Work out the finished part from the listing and answer in its coordinate system (mm). Face numbers are marked on the shaded views. A direction names the side the tool comes from. Coordinates: 2 decimals unless noted, no trailing zeros. Write each loop counter-clockwise with the first axis right and the second up, starting at its lowest first coordinate (ties: lowest second). Pieces come first, ordered by that corner, then holes. Notation, with made-up numbers: (65, 71.5) - (77, 71.5) arc R30 ccw to (77, 95.5) - close; hole circle Ø9 at (45.25, -37). An arc over 180 degrees is marked (long way). Use CSV: the item, a comma, the result in double quotes. Start each with the question number.
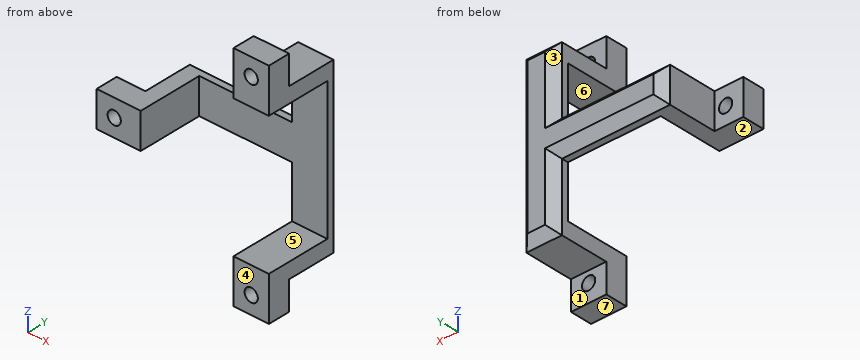
from build123d import *

# Parameters (mm, degrees)
IZIM1_W                       = 10
IZIM1_H                       = 8
IZIM1_R                       = 1.5
Y_KSEKLIK_EKSTR_ZYON1_DEPTH   = 5
IZIM1_W_2                     = 8
IZIM1_H_2                     = 10
Y_KSEKLIK_EKSTR_ZYON1_2_DEPTH = 5
Y_KSEKLIK_EKSTR_ZYON1_3_DEPTH = 5
IZIM2_W                       = 3.5
IZIM2_H                       = 8
IZIM2_W_2                     = 8
IZIM2_H_2                     = 3.5
Y_KSEKLIK_EKSTR_ZYON2_DEPTH   = 13
IZIM3_W                       = 8
IZIM3_H                       = 3.5
Y_KSEKLIK_EKSTR_ZYON3_DEPTH   = 29
IZIM4_W                       = 8
IZIM4_H                       = 3.5
Y_KSEKLIK_EKSTR_ZYON4_DEPTH   = 11.75
IZIM5_W                       = 8
IZIM5_H                       = 3.5
Y_KSEKLIK_EKSTR_ZYON5_DEPTH   = 11.75
PAH1_SIZE                     = 2


with BuildPart() as part:
    # izim1 → Y_kseklik-Ekstr_zyon1 (new body)
    with BuildSketch(Plane(origin=(0, 0, 0), x_dir=(1, 0, 0), z_dir=(0, 1, 0))):
        with Locations((-30, 0)):
            Rectangle(IZIM1_W, IZIM1_H)
        with Locations(Location((-31, 0, 0), (0, 0, 270))):
            Circle(IZIM1_R, mode=Mode.SUBTRACT)
    extrude(amount=Y_KSEKLIK_EKSTR_ZYON1_DEPTH)



with BuildPart() as body_2:
    # izim1 → Y_kseklik-Ekstr_zyon1 2 (new body)
    with BuildSketch(Plane(origin=(0, 0, 0), x_dir=(1, 0, 0), z_dir=(0, 1, 0))):
        with Locations((0, 20.75)):
            Rectangle(IZIM1_W_2, IZIM1_H_2)
        with Locations(Location((0, 21.75, 0), (0, 0, 270))):
            Circle(IZIM1_R, mode=Mode.SUBTRACT)
    extrude(amount=Y_KSEKLIK_EKSTR_ZYON1_2_DEPTH)


with BuildPart() as body_3:
    # izim1 → Y_kseklik-Ekstr_zyon1 3 (new body)
    with BuildSketch(Plane(origin=(0, 0, 0), x_dir=(1, 0, 0), z_dir=(0, 1, 0))):
        with Locations((0, -20.75)):
            Rectangle(IZIM1_W_2, IZIM1_H_2)
        with Locations(Location((0, -21.75, 0), (0, 0, 270))):
            Circle(IZIM1_R, mode=Mode.SUBTRACT)
    extrude(amount=Y_KSEKLIK_EKSTR_ZYON1_3_DEPTH)


with BuildPart() as part_1:
    add(part.part)

    add(body_2.part)  # Y_kseklik-Ekstr_zyon2 merges body 2

    add(body_3.part)  # Y_kseklik-Ekstr_zyon2 merges body 3
    # izim2 → Y_kseklik-Ekstr_zyon2 (add)
    with BuildSketch(Plane(origin=(0, 5, 0), x_dir=(1, 0, 0), z_dir=(0, 1, 0))):
        with Locations((-26.75, 0)):
            Rectangle(IZIM2_W, IZIM2_H)
        with Locations((0, 17.5)):
            Rectangle(IZIM2_W_2, IZIM2_H_2)
        with Locations((0, -17.5)):
            Rectangle(IZIM2_W_2, IZIM2_H_2)
    extrude(amount=Y_KSEKLIK_EKSTR_ZYON2_DEPTH)

    # izim3 → Y_kseklik-Ekstr_zyon3 (add)
    with BuildSketch(Plane(origin=(-25, 0, 0), x_dir=(0, 0, -1), z_dir=(1, 0, 0))):
        with Locations((0, 16.25)):
            Rectangle(IZIM3_W, IZIM3_H)
    extrude(amount=Y_KSEKLIK_EKSTR_ZYON3_DEPTH)

    # izim4 → Y_kseklik-Ekstr_zyon4 (add)
    with BuildSketch(Plane.XY.offset(-15.75)):
        with Locations((0, 16.25)):
            Rectangle(IZIM4_W, IZIM4_H)
    extrude(amount=Y_KSEKLIK_EKSTR_ZYON4_DEPTH)

    # izim5 → Y_kseklik-Ekstr_zyon5 (add)
    with BuildSketch(Plane(origin=(0, 0, 15.75), x_dir=(-1, 0, 0), z_dir=(0, 0, -1))):
        with Locations((0, 16.25)):
            Rectangle(IZIM5_W, IZIM5_H)
    extrude(amount=Y_KSEKLIK_EKSTR_ZYON5_DEPTH)

    # Pah1
    pah1_edges = [part_1.edges().sort_by_distance(p)[0] for p in [
        (-4, 18, 11.625),
        (0, 18, 19.25),
        (4, 18, 0),
        (-4, 18, -11.625),
        (-16.25, 18, -4),
        (-28.5, 18, 0),
        (-16.25, 18, 4),
        (0, 18, -19.25),
    ]]
    chamfer(pah1_edges, length=PAH1_SIZE)


solid = part_1.part
Item 1: A cutting plane is placed at D-D (x = -31). Determine the outline of the cut face in (y, z), then the cut area to 3 significant figures.
Item 2: A cutting plane is placed at B-B (y = 10.75). Determine the outline of the cut face in (x, z).
Item 3: Which of the six approach directions +Z, -Z, +X, -X, +Y, -Y give full straight-line access (tool end or side, diameter ignored) to the marked faces 1, 2 and 3?
Item 4: A cutting plane is placed at A-A (z = 21.75). Determine the outline of the cut face in (x, y), then the cut area to 3 significant figures.
Item 5: Determine the mould class of the marked faces 4, 5, 6 and 7 for opening direction Z: +Z half, -Z half, draft (parallel to the pull), parting line (faces both ways), or undercut.
Item 6: A cutting plane is placed at C-C (x = 0). Determine the outline of the cut face in (y, z).
Item 7: Straight lines are drawn through the part: probe 1 along Z at (x, y) = (-3, 8); probe 2 along X at (y, z) = (3.9, 0); probe 3 along Y at (x, z) = (-0.5, 6). For each, find the intervals that lie inside material, in ascending order. Write a range as [from, to].
Item 8: Each of these flat-tipped pins is pushed along its axis until it touches: pin 1 (7 mm diameter, centred on x = -1, z = -23.5, fed in from +Y); pin 2 (1.5 mm diameter, centred on y = 6, z = 18, fed in from -X); pin 3 (4 mm diameter, centred on x = -7.5, y = 14, fed in from -Z); pin 4 (5 mm diameter, centred on x = -31, z = 0, fed in from -Y). Where does it stop, or does it pass through?
Calculated:
1,outline,"(0, -4) - (5, -4) - (5, -1.5) - (0, -1.5) - close; (0, 1.5) - (5, 1.5) - (5, 4) - (0, 4) - close"
1,area,"25.0 mm²"
2,outline,"(-28.5, -4) - (-25, -4) - (-25, 4) - (-28.5, 4) - close; (-4, -19.25) - (4, -19.25) - (4, -15.75) - (-4, -15.75) - close; (-4, 15.75) - (4, 15.75) - (4, 19.25) - (-4, 19.25) - close"
3,face 1,"-Z, +X, -X, +Y"
3,face 2,"-Z, -X, +Y, -Y"
3,face 3,"+Z, -X, +Y"
4,outline,"(-4, 0) - (-1.5, 0) - (-1.5, 5) - (-4, 5) - close; (1.5, 0) - (4, 0) - (4, 5) - (1.5, 5) - close"
4,area,"25.0 mm²"
5,face 4,"draft"
5,face 5,"undercut"
5,face 6,"undercut"
5,face 7,"-Z half"
6,outline,"(0, -25.75) - (5, -25.75) - (5, -23.25) - (0, -23.25) - close; (0, -20.25) - (5, -20.25) - (5, -19.25) - (16, -19.25) - (18, -17.25) - (18, 17.25) - (16, 19.25) - (5, 19.25) - (5, 20.25) - (0, 20.25) - (0, 15.75) - (14.5, 15.75) - (14.5, -15.75) - (0, -15.75) - close; (0, 23.25) - (5, 23.25) - (5, 25.75) - (0, 25.75) - close"
7,probe 1,"z = [-19.25, -15.75], [15.75, 19.25]"
7,probe 2,"x = [-35, -32.5], [-29.5, -25]"
7,probe 3,"y = [14.5, 18]"
8,pin 1,"stops at y = 5"
8,pin 2,"stops at x = -4"
8,pin 3,"stops at z = -4"
8,pin 4,"stops at y = 0"
